Part model, mm, in its own coordinate system. Face numbers are marked on the shaded views. A direction names the side the tool comes from. Give positions to 0.01 mm unless a question says otherwise; leave off trailing zeros. Order: outer loops, then holes, each group sorted by start corner. A loop starts at its lowest first (then second) coordinate and runs counter-clockwise, first axis right, second up. Notation, with made-up numbers: (77.5, -21) -> (114.5, -21) arc R27 cw to (114.5, 3) -> close; hole circle Ø11 at (1.25, 85). An arc over 180 degrees is marked (long way). Write item = value, one per line. Start each with the question number.
(1) Which spindle directions (+Z, -Z, +X, -X, +Y, -Y) get a long thin tool onto all of the face, cutting with end or side? Do the marked faces 1, 2 and 3. Say none if no direction does.
(2) Saw through at D-D, the plane z = -4.5. List the corners of the cut face in (x, y), then the cut area to 3 significant figures.
(3) Saw through at A-A, the plane y = 11. List the corners of the cut face in (x, z).
(4) Two-plate mould, pull along Y, no slides. Class the marked faces 4, 5, 6 and 7: pulls with the +Y half, pulls with the -Y half, needs draft (parallel to the pull), parting line crosses it, or undercut.
(5) Flat gauge pins, fed straight in: pin 1 (1.5 mm diameter, centred on y = 8, z = -2, fed in from -X); pin 2 (1.2 mm diameter, centred on y = 1.5, z = -1, fed in from +X). Where does each tip first touch, or does it go through?
(6) Saw through at B-B, the plane x = -0.5. List the corners of the cut face in (y, z).
(7) Probe line 1 along Z through (x, y) = (-2.55, 11); line 2 along X through (y, z) = (12, 5.75); line 3 along X through (y, z) = (1, 2.25). List the from-to ranges inside material, lowest first. Write a range as from..to.
(8) Saw through at C-C, the plane z = 0. List the corners of the cut face in (x, y), then the cut area to 3 significant figures.
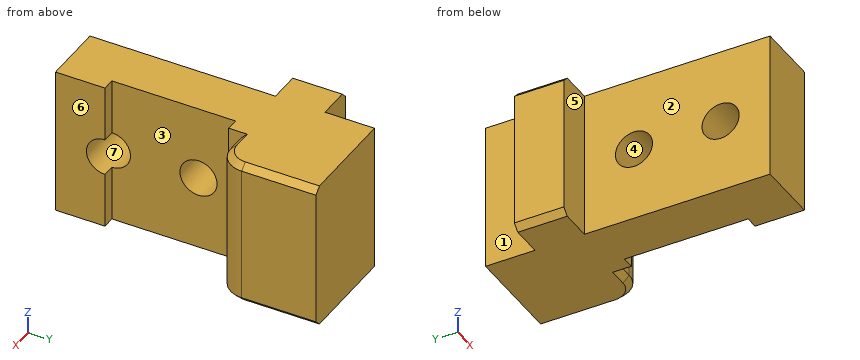
Autodesk Inventor part; units mm, degrees
ref_plane "YZ Plane" through (0, 0, 0) normal (1, 0, 0) x (0, 1, 0)
ref_plane "XZ Plane" through (0, 0, 0) normal (0, 1, 0) x (-1, 0, 0)
ref_plane "XY Plane" through (0, 0, 0) normal (0, 0, 1) x (1, 0, 0)
sketch "Sketch1" plane through (0, 0, 0) normal (0, 0, 1) x (1, 0, 0)
  line L0 (0, 0) -> (0, 4)
  line L1 (0, 4) -> (-1, 4)
  line L2 (-1, 4) -> (-1, 14)
  line L3 (-1, 14) -> (0, 14)
  line L4 (0, 14) -> (0, 15)
  line L5 (0, 15) -> (1.5, 15)
  line L6 (3.5, 17) -> (3.5, 23)
  line L7 (3.5, 23) -> (-5, 23)
  line L8 (-5, 23) -> (-5, 19)
  line L9 (-5, 19) -> (-8, 19)
  line L10 (-8, 19) -> (-8, 15)
  line L11 (-8, 15) -> (-5, 15)
  line L12 (-5, 15) -> (-5, 0)
  line L13 (-5, 0) -> (0, 0)
  arc A0 (1.5, 15) -> (3.5, 17) centre (1.5, 17) ccw
  point P0 (0.75, 15)
  point P1 (-0.5, 4)
  point P2 (0, 2)
  point P3 (-6.5, 15)
  point P4 (-6.5, 19)
  point P5 (-5, 21)
  dimension "d3" = 4
  dimension "d4" = 14
  dimension "d6" = 1
  dimension "d7" = 1
  dimension "d8" = 5
  dimension "d9" = 8
  dimension "d10" = 3
  dimension "d12" = 0
  dimension "d13" = 4
  dimension "d14" = 2
  dimension "d15" = 8.5
  dimension "d16" = 5
extrude "Extrusion1" add sketch "Sketch1" along normal mid plane 12
chamfer "Chamfer1" distance 0.5 angle 45 8 edges at (3.5, 20, 6) (2.9142, 15.5858, 6) (0.75, 15, 6) (-8, 17, 6) (3.5, 20, -6) (2.9142, 15.5858, -6) (0.75, 15, -6) (-8, 17, -6)
sketch "Sketch2" plane through (0, 0, 0) normal (1, 0, 0) x (0, 1, 0)
  circle A0 centre (4, 0) radius 1.5
  circle A1 centre (11, 0) radius 1.5
  line L0 (14, -6) -> (14, 6)
  line L1 (0, -6) -> (0, 6)
  point P0 (0, 0)
  point P1 (0, 0)
  point P2 (0, 0)
  dimension "d22" = 3
  dimension "d23" = 3
  dimension "d24" = 7
  dimension "d25" = 3
  dimension "d26" = 0
  dimension "d27" = 0
extrude "Extrusion2" cut sketch "Sketch2" against normal through all
properties part number "connector"
Results list:
q1.face_1 = +Z, -Z, -X, +Y
q1.face_2 = +Z, -Z, -X, -Y
q1.face_3 = +Z, -Z, +X
q2.outline = (-8, 15) -> (-5, 15) -> (-5, 0) -> (0, 0) -> (0, 4) -> (-1, 4) -> (-1, 14) -> (0, 14) -> (0, 15) -> (1.5, 15) arc R2 ccw to (3.5, 17) -> (3.5, 23) -> (-5, 23) -> (-5, 19) -> (-8, 19) -> close
q2.area = 144 mm^2
q3.outline = (-5, -6) -> (-1, -6) -> (-1, -1.5) -> (-5, -1.5) -> close; (-5, 1.5) -> (-1, 1.5) -> (-1, 6) -> (-5, 6) -> close
q4.face_4 = undercut
q4.face_5 = pulls with the -Y half
q4.face_6 = needs draft
q4.face_7 = undercut
q5.pin_1 = -5
q5.pin_2 = 0
q6.outline = (0, -6) -> (4, -6) -> (4, -1.5) arc R1.5 cw to (4, 1.5) -> (4, 6) -> (0, 6) -> close; (14, -6) -> (23, -6) -> (23, 6) -> (14, 6) -> close
q7.line_1 = -6..-1.5, 1.5..6
q7.line_2 = -5..-1
q7.line_3 = -5..0
q8.outline = (-8, 15) -> (-5, 15) -> (-5, 12.5) -> (-1, 12.5) -> (-1, 14) -> (0, 14) -> (0, 15) -> (1.5, 15) arc R2 ccw to (3.5, 17) -> (3.5, 23) -> (-5, 23) -> (-5, 19) -> (-8, 19) -> close; (-5, 0) -> (0, 0) -> (0, 2.5) -> (-5, 2.5) -> close; (-5, 5.5) -> (-1, 5.5) -> (-1, 9.5) -> (-5, 9.5) -> close
q8.area = 119 mm^2
